```python
from build123d import *

# Parameters (mm, degrees)
ESBO_O1_R                        = 4
RESSALTO_EXTRUS_O1_DEPTH         = 16
ESBO_O2_R                        = 3.5
RESSALTO_EXTRUS_O2_DEPTH         = 1.95
ESBO_O4_R                        = 1.95
RESSALTO_EXTRUS_O4_DEPTH         = 0.9
ESBO_O5_R                        = 0.5
RESSALTO_EXTRUS_O5_DEPTH         = 2.5
ESBO_O6_W                        = 1.8
ESBO_O6_H                        = 0.15
RESSALTO_EXTRUS_O6_DEPTH         = 4.1
CHANFRO1_SIZE                    = 0.5
CORTE_EXTRUS_O1_REACH            = 21.667
ESBO_O7_W                        = 1.6
ESBO_O7_H                        = 1
PADR_OCIRCULAR1_COUNT            = 2
CHANFRO1_OF_PADR_OCIRCULAR1_SIZE = 0.5
ESBO_O3_R                        = 1.55
CORTE_EXTRUS_O2_DEPTH            = 0.65
RESSALTO_EXTRUS_O7_START         = 4.2
ESBO_O9_R                        = 0.5
RESSALTO_EXTRUS_O7_DEPTH         = 4.2


with BuildPart() as part:
    # Esboço1 → Ressalto-extrusão1 (new body)
    with BuildSketch(Plane(origin=(0, 0, 0), x_dir=(0, 0, -1), z_dir=(1, 0, 0))):
        Circle(ESBO_O1_R)
    extrude(amount=-RESSALTO_EXTRUS_O1_DEPTH)

    # Esboço2 → Ressalto-extrusão2 (add)
    with BuildSketch(Plane.ZY.offset(16)):
        Circle(ESBO_O2_R)
    extrude(amount=RESSALTO_EXTRUS_O2_DEPTH)

    # Esboço4 → Ressalto-extrusão4 (add)
    with BuildSketch(Plane(origin=(0, 0, 0), x_dir=(0, 0, -1), z_dir=(1, 0, 0))):
        Circle(ESBO_O4_R)
    extrude(amount=RESSALTO_EXTRUS_O4_DEPTH)

    # Esboço5 → Ressalto-extrusão5 (add)
    with BuildSketch(Plane(origin=(0.9, 0, 0), x_dir=(0, 0, -1), z_dir=(1, 0, 0))):
        Circle(ESBO_O5_R)
    extrude(amount=RESSALTO_EXTRUS_O5_DEPTH)

    # Esboço6 → Ressalto-extrusão6 (add)
    with BuildSketch(Plane(origin=(0, 0, 0), x_dir=(0, 0, -1), z_dir=(1, 0, 0))):
        with Locations((0, 2.896690855)):
            Rectangle(ESBO_O6_W, ESBO_O6_H)
    ressalto_extrus_o6 = extrude(amount=RESSALTO_EXTRUS_O6_DEPTH)

    # Chanfro1
    chanfro1_edges = [part.edges().sort_by_distance(p)[0] for p in [
        (4.1, 2.896690855, 0.9),
        (4.1, 2.896690855, -0.9),
    ]]
    chamfer(chanfro1_edges, length=CHANFRO1_SIZE)

    # Esboço7 → Corte-extrusão1 (cut, up to next)
    with BuildSketch(Plane(origin=(0, 2.971690855, 0), x_dir=(1, 0, 0), z_dir=(0, 1, 0)), mode=Mode.PRIVATE) as corte_extrus_o1_sk1:
        with Locations((2.9, 0)):
            Rectangle(ESBO_O7_W, ESBO_O7_H)
    corte_extrus_o1_tool1 = extrude(corte_extrus_o1_sk1.sketch, amount=-CORTE_EXTRUS_O1_REACH, mode=Mode.PRIVATE) & part.part
    corte_extrus_o1 = corte_extrus_o1_tool1.solids().sort_by_distance((2.9, 2.971691, 0))[0]
    add(corte_extrus_o1, mode=Mode.SUBTRACT)

    # PadrãoCircular1: Ressalto-extrusão6, Corte-extrusão1 ×2 about axis
    padr_ocircular1_axis = Axis((0, 0, 0), (1, 0, 0))
    add([ressalto_extrus_o6.rotate(padr_ocircular1_axis, i * 360 / PADR_OCIRCULAR1_COUNT) for i in range(1, PADR_OCIRCULAR1_COUNT)])
    add([corte_extrus_o1.rotate(padr_ocircular1_axis, i * 360 / PADR_OCIRCULAR1_COUNT) for i in range(1, PADR_OCIRCULAR1_COUNT)], mode=Mode.SUBTRACT)

    # Chanfro1 of PadrãoCircular1
    chanfro1_of_padr_ocircular1_edges = [part.edges().sort_by_distance(p)[0] for p in [
        (4.1, -2.896690855, -0.9),
        (4.1, -2.896690855, 0.9),
    ]]
    chamfer(chanfro1_of_padr_ocircular1_edges, length=CHANFRO1_OF_PADR_OCIRCULAR1_SIZE)

    # Esboço3 → Corte-extrusão2 (cut)
    with BuildSketch(Plane.ZY.offset(17.95)):
        Circle(ESBO_O3_R)
    extrude(amount=-CORTE_EXTRUS_O2_DEPTH, mode=Mode.SUBTRACT)

    # Esboço9 → Ressalto-extrusão7 (add)
    with BuildSketch(Plane.ZY.offset(17.3).offset(RESSALTO_EXTRUS_O7_START)):
        with Locations(Location((0, 0, 0), (0, 0, 180))):
            Circle(ESBO_O9_R)
    extrude(amount=-RESSALTO_EXTRUS_O7_DEPTH)


solid = part.part
```
Geometry check sheet. Reference: the model listing, model coordinates, mm. A direction names the side the tool comes from. Coordinates: 2 decimals unless noted, no trailing zeros. Order: outer loops, then holes, each group sorted by start corner. A loop starts at its lowest first (then second) coordinate and runs counter-clockwise, first axis right, second up. Notation, with made-up numbers: (87.25, -25.75) - (143.25, -25.75) arc R22 ccw to (143.25, 6.25) - close; hole circle Ø4 at (88, 84). An arc over 180 degrees is marked (long way). Answer in a Markdown table with one row per item. Add a question column.
1. Section check D-D (x = -19.5). Enter the section's corners in (y, z).
2. Material ranges on L1, parallel to Y at x = -17.6, z = 0; L2, parallel to X at y = 1.5, z = -3.5; L3, parallel to X at y = 1.75, z = 0.75, recorded low to high. Write a range as [from, to].
3. Gauge pin test, flat ends, axial feed: pin 1 Ø3 at (x, z) = (-1, 2.5) entering from -Y; pin 2 Ø2 at (y, z) = (3, 0.5) entering from -X; pin 3 Ø0.9 at (x, z) = (2.5, 0) entering from -Y. Record the tip position at first contact, or that the pin passes through.
4. Section check A-A (x = 1.5). Enter the section's corners in (y, z).
5. Section check C-C (z = 0). Give the number of separate pieces and of enclosed holes in the cut face, plus the area to 3 significant figures.
6. Access from +Z, -Z, +X, -X, +Y, -Y to the whole of each face (thin tool, end or side, straight path). Record for faces 1 (the face through (2.132, -0.488, 0.108)), 2 (the face through (-19.429, 0.488, 0.108)), 3 (the face through (1.6, -2.972, 0)), 4 (the face through (1.6, 2.972, 0)).
7. Section check B-B (y = 0). Enter the section's corners in (x, z).
8. Draft check along Z on faces 5 (the face through (-7.888, -3.905, 0.867)), 6 (the face through (-17.63, -1.375, 0.715)), 7 (the face through (-17.95, -2, 1)). Enter one of: +Z half, -Z half, draft (parallel to the pull), parting line (faces both ways), or undercut.
Data:
| question | item | result |
|---|---|---|
| 1 | outline | circle Ø1 at (0, 0) |
| 2 | L1 | y = [-3.5, -1.55], [-0.5, 0.5], [1.55, 3.5] |
| 2 | L2 | x = [-16, 0] |
| 2 | L3 | x = [-17.95, 0.9] |
| 3 | pin 1 | stops at y = -3.87 |
| 3 | pin 2 | stops at x = -17.95 |
| 3 | pin 3 | stops at y = -2.97 |
| 4 | outline | (-2.97, -0.9) - (-2.82, -0.9) - (-2.82, 0.9) - (-2.97, 0.9) - close; circle Ø1 at (0, 0); (2.82, -0.9) - (2.97, -0.9) - (2.97, 0.9) - (2.82, 0.9) - close |
| 5 | separate pieces | 3 |
| 5 | enclosed holes | 0 |
| 5 | area | 151 mm² |
| 6 | face 1 | +X |
| 6 | face 2 | -X |
| 6 | face 3 | +Z, -Z, +X, -Y |
| 6 | face 4 | +Z, -Z, +X, +Y |
| 7 | outline | (-21.5, -0.5) - (-17.3, -0.5) - (-17.3, -1.55) - (-17.95, -1.55) - (-17.95, -3.5) - (-16, -3.5) - (-16, -4) - (0, -4) - (0, -1.95) - (0.9, -1.95) - (0.9, -0.5) - (3.4, -0.5) - (3.4, 0.5) - (0.9, 0.5) - (0.9, 1.95) - (0, 1.95) - (0, 4) - (-16, 4) - (-16, 3.5) - (-17.95, 3.5) - (-17.95, 1.55) - (-17.3, 1.55) - (-17.3, 0.5) - (-21.5, 0.5) - close |
| 8 | face 5 | parting line |
| 8 | face 6 | undercut |
| 8 | face 7 | draft |
